Source: CAD feature listing. Evaluate the final solid. Frame: model axes, mm. A direction names the side the tool comes from. Give positions to 0.01 mm unless a question says otherwise; leave off trailing zeros. Loops run counter-clockwise (first coordinate to the right, second up) from the corner with the lowest first, then second, coordinate; pieces in that order, holes last. Notation, with made-up numbers: M 44.25,40.5 L 81.25,40.5 A11 ccw 81.25,48.5 Z; hole C 64,-19 d6. An arc over 180 degrees is marked long. Answer in a Markdown table with one row per item.
```python
from build123d import *

# Parameters (mm, degrees)
SKETCH1_R           = 1.15
BOSS_EXTRUDE1_DEPTH = 0.2
SKETCH2_W           = 11.2
SKETCH2_H           = 5.8
BOSS_EXTRUDE2_DEPTH = 5
SKETCH3_W           = 3
SKETCH3_H           = 3
BOSS_EXTRUDE3_DEPTH = 5.5


with BuildPart() as part:
    # Sketch1 → Boss-Extrude1 (new body)
    with BuildSketch(Plane(origin=(0, 0, 0), x_dir=(1, 0, 0), z_dir=(0, 1, 0))):
        Polygon((9.5, 2.325), (9.5, -2.325), (5.6, -2.325), (5.6, -2.9), (-5.6, -2.9), (-5.6, -2.325), (-9.5, -2.325), (-9.5, 2.325), (-5.6, 2.325), (-5.6, 2.9), (5.6, 2.9), (5.6, 2.325), align=None)
        with Locations(Location((-7.75, 0, 0), (0, 0, 270))):
            Circle(SKETCH1_R, mode=Mode.SUBTRACT)
        with Locations(Location((7.75, 0, 0), (0, 0, 270))):
            Circle(SKETCH1_R, mode=Mode.SUBTRACT)
    extrude(amount=BOSS_EXTRUDE1_DEPTH)

    # Sketch2 → Boss-Extrude2 (add)
    with BuildSketch(Plane.XZ):
        Rectangle(SKETCH2_W, SKETCH2_H)
    extrude(amount=BOSS_EXTRUDE2_DEPTH)

    # Sketch3 → Boss-Extrude3 (add)
    with BuildSketch(Plane(origin=(0, 0.2, 0), x_dir=(1, 0, 0), z_dir=(0, 1, 0))):
        Rectangle(SKETCH3_W, SKETCH3_H)
    extrude(amount=BOSS_EXTRUDE3_DEPTH)


solid = part.part
```
Q1. Section query B-B (z = 0). Output: boundary loops of the cut face in (x, y).
Values follow:
| item | result |
|---|---|
| outline | M -9.5,0 L -8.9,0 L -8.9,0.2 L -9.5,0.2 Z; M -6.6,0 L -5.6,0 L -5.6,-5 L 5.6,-5 L 5.6,0 L 6.6,0 L 6.6,0.2 L 1.5,0.2 L 1.5,5.7 L -1.5,5.7 L -1.5,0.2 L -6.6,0.2 Z; M 8.9,0 L 9.5,0 L 9.5,0.2 L 8.9,0.2 Z |
Q2. Section query D-D (y = -3.25). Output: boundary loops of the cut face in (x, z).
Values follow:
| item | result |
|---|---|
| outline | M -5.6,-2.9 L 5.6,-2.9 L 5.6,2.9 L -5.6,2.9 Z |
Q3. Contact query for flat-ended pins moving along their axis: pin 1 Ø2.5 at (y, z) = (-2, -1.5) entering from -X; pin 2 Ø3 at (x, z) = (-8, 0) entering from -Y; pin 3 Ø2.5 at (x, y) = (0.5, 4) entering from -Z. Output: stop coordinate, or through.
Values follow:
| item | result |
|---|---|
| pin 1 | x = -5.6 |
| pin 2 | y = 0 |
| pin 3 | z = -1.5 |
Q4. Section query A-A (x = 7.75). Output: boundary loops of the cut face in (y, z) (3 decimals).
Values follow:
| item | result |
|---|---|
| outline | M 0,-2.325 L 0.2,-2.325 L 0.2,-1.15 L 0,-1.15 Z; M 0,1.15 L 0.2,1.15 L 0.2,2.325 L 0,2.325 Z |
Q5. Reachability of faces 1 (the flat face through (1.5, 3, 0)), 2 (the flat face through (0, 3, 1.5)), 3 (the flat face through (-1.5, 3, 0)), 4 (the flat face through (0, 3, -1.5)) from +Z, -Z, +X, -X, +Y, -Y: full face, straight path, thin tool, end or side. Return the list, or none.
Values follow:
| item | result |
|---|---|
| face 1 | +Z, -Z, +X, +Y |
| face 2 | +Z, +X, -X, +Y |
| face 3 | +Z, -Z, -X, +Y |
| face 4 | -Z, +X, -X, +Y |
Q6. Section query C-C (x = 0.75). Output: boundary loops of the cut face in (y, z), plus the area to 3 significant figures.
Values follow:
| item | result |
|---|---|
| outline | M -5,-2.9 L 0.2,-2.9 L 0.2,-1.5 L 5.7,-1.5 L 5.7,1.5 L 0.2,1.5 L 0.2,2.9 L -5,2.9 Z |
| area | 46.7 mm^2 |
Q7. Ray query, probe 1 along X at (y, z) = (0.1, 0); probe 2 along Y at (x, z) = (3.25, -0.6); probe 3 along X at (y, z) = (-3.5, 0.7). Return the intervals inside material, ascending. Write a range as from..to.
Values follow:
| item | result |
|---|---|
| probe 1 | -9.5..-8.9, -6.6..6.6, 8.9..9.5 |
| probe 2 | -5..0.2 |
| probe 3 | -5.6..5.6 |
